```python
from build123d import *

# Parameters (mm, degrees)
F1_DEPTH = 6.35
F1_TAPER = 22.5
F2_R     = 12.7
F3_DEPTH = 3.175
F4_R     = 3.175
F5_DEPTH = 25.4


with BuildPart() as f1:
    # F0 (on Top) → F1 (new body)
    with BuildSketch(Plane.XY):
        Polygon((-30.9957823292, 12.7266398535), (-30.9164212153, -12.9182345311), (-12.7266398535, -30.9957823292), (12.9182345311, -30.9164212153), (30.9957823292, -12.7266398535), (30.9164212153, 12.9182345311), (12.7266398535, 30.9957823292), (-12.9182345311, 30.9164212153), align=None)
    extrude(amount=-F1_DEPTH, taper=F1_TAPER)

    # F2 (on face) → F3 (cut)
    with BuildSketch(Plane.XY):
        Circle(F2_R)
    extrude(amount=-F3_DEPTH, mode=Mode.SUBTRACT)

    # F4 (on face) → F5 (cut)
    with BuildSketch(Plane.XY.offset(-3.175)):
        Circle(F4_R)
    extrude(amount=-F5_DEPTH, mode=Mode.SUBTRACT)


solid = f1.part
```
Could you check a few things on this model? Use its own coordinates, in mm. A direction names the side the tool comes from. Coordinates: 2 decimals unless noted, no trailing zeros. Use one line per item in the form item = value. Start each with the question number.
1. We'd pull the mould along Y, two halves only. Please class faces 3 (the flat face through (5, 14, 0)), 4 (the flat face through (3, -3, -3.175)): +Y half, -Y half, draft (parallel to the pull), parting line (faces both ways), or undercut.
2. On a 3-axis mill with a long thin cutter (end or side, diameter ignored), from which of +Z, -Z, +X, -X, +Y, -Y can I reach the whole of each face in a straight line? I mean faces 1 (the flat face through (2, 6, -6.35)), 2 (the cylindrical face through (-2.75, -12.4, -1.57)). Say none if no direction works.
3. For pin 1 (5 mm diameter, centred on x = 0, y = 0, fed in from -Z); pin 2 (2 mm diameter, centred on y = 22.5, z = -3, fed in from -X); pin 3 (1.5 mm diameter, centred on y = -22.5, z = -2, fed in from -X); pin 4 (1.5 mm diameter, centred on x = -8.5, z = -2.5, fed in from +Y), each with a flat end and sliding along its axis, tell me the tip position at first contact or that it passes through.
4. Please list where these lines run through material, in increasing order: line 1 (X direction, y = -5.5, z = -1.25); line 2 (X direction, y = 4.5, z = -0.75); line 3 (Y direction, x = 0, z = -2).
Geometry says:
q1.face_3 = draft
q1.face_4 = undercut
q2.face_1 = -Z, +X, -X, +Y, -Y
q2.face_2 = +Z
q3.pin_1 = through
q3.pin_2 = -20.68
q3.pin_3 = -20.97
q3.pin_4 = 30.21
q4.line_1 = -30.42 to -11.45, 11.45 to 30.46
q4.line_2 = -30.66 to -11.88, 11.88 to 30.63
q4.line_3 = -30.13 to -12.7, 12.7 to 30.13
